Can you work these out from the model? Positions are in its coordinate system, mm. Coordinates: 2 decimals unless noted, no trailing zeros. Order: outer loops, then holes, each group sorted by start corner. A loop starts at its lowest first (then second) coordinate and runs counter-clockwise, first axis right, second up. Notation, with made-up numbers: (-15, 63) -> (19, 63) arc R15 cw to (19, 85) -> close; hole circle Ø11 at (68.25, 72). An arc over 180 degrees is marked (long way). Use a Markdown table: item, result. Add a question column.
1. Suppose I cut it at A-A, the plane z = 2.35. State how many separate pieces and enclosed holes the cut face has, then the cut area to 3 significant figures.
2. Suppose I cut it at D-D, the plane y = -40. List the corners of the cut face in (x, z) for me, then the cut area to 3 significant figures.
3. For pin 1 Ø1.8 at (x, y) = (110, 0) entering from +Z; pin 2 Ø2 at (x, z) = (111.5, 4.5) entering from +Y; pin 3 Ø1.5 at (y, z) = (-5, 1.5) entering from +X; pin 4 Ø1.5 at (x, z) = (-17, 4) entering from +Y, each with a flat end and sliding along its axis, tell me the tip position at first contact or that it passes through.
4. If I drill on line 1 along Y through (x, z) = (0, 3.2); line 2 along X through (y, z) = (2.5, 3.75); line 3 along X through (y, z) = (3, 2.15), over which ranges is the centre line in solid material (lowest first)? Write a range as from..to.
5. We'd pull the mould along Y, two halves only. Please class faces 1 (the flat face through (32, 1, 0)), 2 (the flat face through (82.174, -34.272, 2.465)), 3 (the cylindrical face through (-0.867, -3.905, 2.465)): pulls with the +Y half, pulls with the -Y half, needs draft (parallel to the pull), parting line crosses it, or undercut.
6. Suppose I cut it at B-B, the plane x = 150. List the corners of the cut face in (y, z) for me, then the cut area to 3 significant figures.
7. Suppose I cut it at C-C, the plane x = 40.5. List the corners of the cut face in (y, z) for me, then the cut area to 3 significant figures.
```python
from build123d import *

# Parameters (mm, degrees)
SKETCH1_R           = 1.5
SKETCH1_R_2         = 4
BOSS_EXTRUDE1_DEPTH = 5


with BuildPart() as part:
    # Sketch1 → Boss-Extrude1 (new body)
    with BuildSketch(Plane.XY):
        with BuildLine():
            ThreePointArc((12.25, 51.05083251), (-52.5, 0), (12.25, -51.05083251))
            Line((12.25, -51.05083251), (154.083333333, -17.01694417))
            ThreePointArc((154.083333333, -17.01694417), (167.5, 0), (154.083333333, 17.01694417))
            Line((154.083333333, 17.01694417), (12.25, 51.05083251))
        make_face()
        with Locations((0, -15)):
            Circle(SKETCH1_R, mode=Mode.SUBTRACT)
        with Locations((-15, 0)):
            Circle(SKETCH1_R, mode=Mode.SUBTRACT)
        Circle(SKETCH1_R_2, mode=Mode.SUBTRACT)
        with BuildLine():
            ThreePointArc((16.5, 0), (15, -1.5), (13.5, 0))
            ThreePointArc((13.5, 0), (15, 1.5), (16.5, 0))
        make_face(mode=Mode.SUBTRACT)
        with Locations((0, 15)):
            Circle(SKETCH1_R, mode=Mode.SUBTRACT)
        with Locations((70, 0)):
            Circle(SKETCH1_R, mode=Mode.SUBTRACT)
        with Locations((90, 0)):
            Circle(SKETCH1_R, mode=Mode.SUBTRACT)
        with Locations((110, 0)):
            Circle(SKETCH1_R, mode=Mode.SUBTRACT)
        with Locations((150, 0)):
            Circle(SKETCH1_R_2, mode=Mode.SUBTRACT)
    extrude(amount=BOSS_EXTRUDE1_DEPTH)


solid = part.part
```
Worked out:
| question | item | result |
|---|---|---|
| 1 | separate pieces | 1 |
| 1 | enclosed holes | 9 |
| 1 | area | 15,400 mm² |
| 2 | outline | (-34, 0) -> (58.3, 0) -> (58.3, 5) -> (-34, 5) -> close |
| 2 | area | 462 mm² |
| 3 | pin 1 | passes through |
| 3 | pin 2 | stops at y = 27.48 |
| 3 | pin 3 | stops at x = 166.98 |
| 3 | pin 4 | stops at y = 49.92 |
| 4 | line 1 | y = -52.5..-16.5, -13.5..-4, 4..13.5, 16.5..52.5 |
| 4 | line 2 | x = -52.44..-3.12, 3.12..146.88, 153.12..167.32 |
| 4 | line 3 | x = -52.41..-2.65, 2.65..147.35, 152.65..167.24 |
| 5 | face 1 | needs draft |
| 5 | face 2 | pulls with the -Y half |
| 5 | face 3 | undercut |
| 6 | outline | (-18, 0) -> (-4, 0) -> (-4, 5) -> (-18, 5) -> close; (4, 0) -> (18, 0) -> (18, 5) -> (4, 5) -> close |
| 6 | area | 140 mm² |
| 7 | outline | (-44.27, 0) -> (44.27, 0) -> (44.27, 5) -> (-44.27, 5) -> close |
| 7 | area | 443 mm² |
